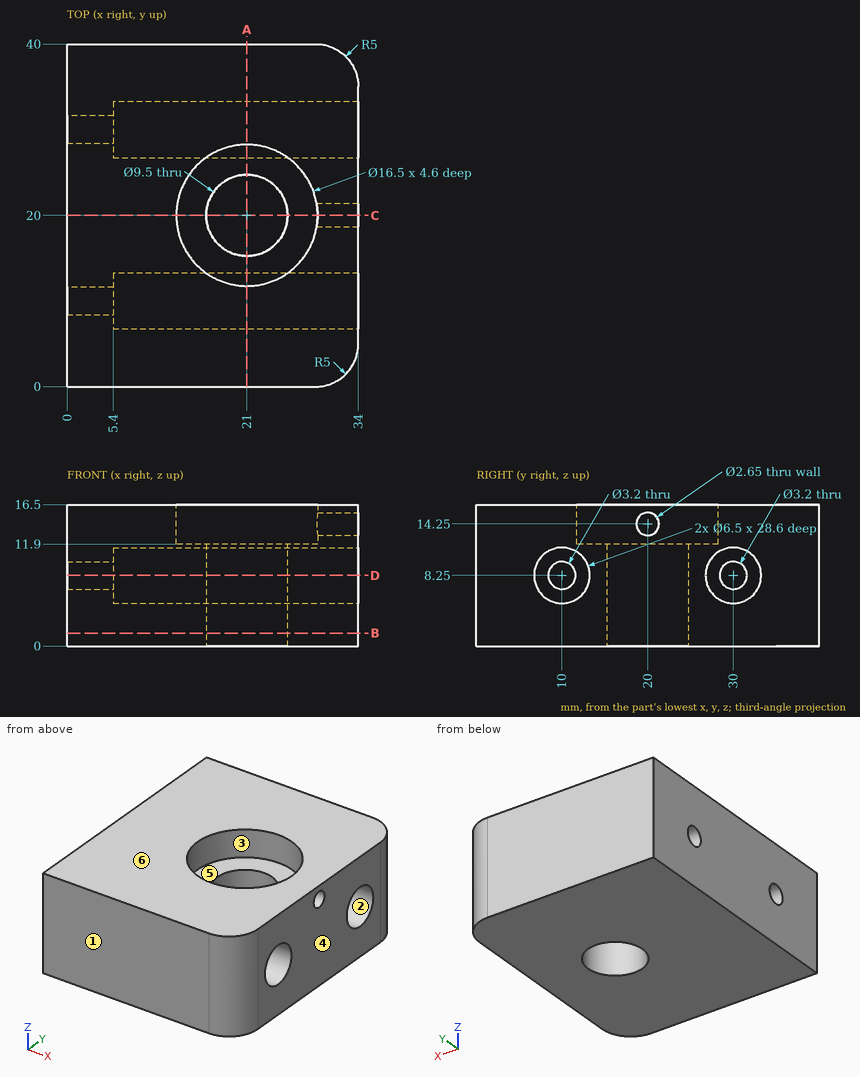
The figure shows three views and two pictorial views of one solid part (mm, origin at its lowest corner). Answer the questions. A direction names the side the tool comes from. Round coordinates to 2 decimals unless told otherwise and drop trailing zeros. Loops run counter-clockwise (first coordinate to the right, second up) from the corner with the lowest first, then second, coordinate; pieces in that order, holes last. Notation, with made-up numbers: M -7,57 L 45,57 A30 ccw 45,95 Z; hole C 1,37.5 d2. An arc over 180 degrees is marked long. Return JSON: item names as keys, results as strings.
Q1. Find the intervals of material crossed by line 1 along Z through (x, y) = (24, 30); line 2 along Z through (x, y) = (32.5, 20) (3 decimals); line 3 along Y through (x, z) = (21, 15.35), in increasing order. Write a range as from..to.
Results list:
{"line 1": "z = 0..5, 11.5..16.5", "line 2": "z = 0..12.925, 15.575..16.5", "line 3": "y = 0..11.75, 28.25..40"}
Q2. Find section C-C, the plane y = 20. Determine the outline of the cut face in (x, z) (3 decimals).
Results list:
{"outline": "M 0,0 L 16.25,0 L 16.25,11.9 L 12.75,11.9 L 12.75,16.5 L 0,16.5 Z; M 25.75,0 L 34,0 L 34,12.925 L 29.25,12.925 L 29.25,11.9 L 25.75,11.9 Z; M 29.25,15.575 L 34,15.575 L 34,16.5 L 29.25,16.5 Z"}
Q3. The mould has two halves that part along X. Classify the marked faces 4, 5 and 6: released by +X, released by -X, zero draft, split by the parting line, or undercut.
Results list:
{"face 4": "released by +X", "face 5": "undercut", "face 6": "zero draft"}
Q4. Find section A-A, the plane x = 21. Determine the outline of the cut face in (y, z), plus the area to 3 significant figures.
Results list:
{"outline": "M 0,0 L 15.25,0 L 15.25,11.9 L 11.75,11.9 L 11.75,16.5 L 0,16.5 Z; M 24.75,0 L 40,0 L 40,16.5 L 28.25,16.5 L 28.25,11.9 L 24.75,11.9 Z; hole C 10,8.25 d6.5; hole C 30,8.25 d6.5", "area": "405 mm2"}
Q5. Find section D-D, the plane z = 8.25. Determine the outline of the cut face in (x, y).
Results list:
{"outline": "M 0,0 L 29,0 A5 ccw 34,5 L 34,6.75 L 5.4,6.75 L 5.4,8.4 L 0,8.4 Z; M 0,11.6 L 5.4,11.6 L 5.4,13.25 L 34,13.25 L 34,26.75 L 5.4,26.75 L 5.4,28.4 L 0,28.4 Z; M 0,31.6 L 5.4,31.6 L 5.4,33.25 L 34,33.25 L 34,35 A5 ccw 29,40 L 0,40 Z; hole C 21,20 d9.5"}
Q6. Which of the six approach directions +Z, -Z, +X, -X, +Y, -Y give full straight-line access (tool end or side, diameter ignored) to the marked faces 1, 2 and 3?
Results list:
{"face 1": "+Z, -Z, +X, -X, -Y", "face 2": "+X", "face 3": "+Z"}
Q7. Each of these flat-tipped pins is pushed along its axis until it touches: pin 1 Ø15 at (x, y) = (21, 20) entering from +Z; pin 2 Ø3 at (y, z) = (10.5, 7) entering from +X. Where does it stop, or does it pass through?
Results list:
{"pin 1": "stops at z = 11.9", "pin 2": "stops at x = 5.4"}
Q8. Find section B-B, the plane z = 1.5. Determine the outline of the cut face in (x, y).
Results list:
{"outline": "M 0,0 L 29,0 A5 ccw 34,5 L 34,35 A5 ccw 29,40 L 0,40 Z; hole C 21,20 d9.5"}
